Here's how the part is built. I have some questions about the finished solid (model axes, mm). A direction names the side the tool comes from. Give positions to 0.01 mm unless a question says otherwise; leave off trailing zeros. Loops run counter-clockwise (first coordinate to the right, second up) from the corner with the lowest first, then second, coordinate; pieces in that order, holes last.
Q1. Suppose I cut it at C-C (y = 219). List the corners of the cut face in (x, z) for me.
Q2. Suppose I cut it at D-D (z = 499). List the corners of the cut face in (x, y) for me.
Q3. Suppose I cut it at B-B (z = -166). List the corners of the cut face in (x, y) for me.
Q4. Thinking about a two-plate mould opening in X: for faces 6 (the face through (789.91, 959.68, -563.82)), 7 (the face through (-419.1, 161, -206)), 8 (the face through (201.28, 927.28, -543.77)), which applies, pulls with the +X half, pulls with the -X half, needs draft (parallel to the pull), parting line crosses it, or undercut?
Q5. I'm going to push flat-ended pins straight in: P1, Ø3, axis at x = -54, y = 900.5, coming from the +Z side; P2, Ø2, axis at x = 529.5, y = 641.5, coming from the +Z side; P3, Ø5, axis at x = 292, y = -83.5, coming from the -Z side. Where does each tip first touch, or does it pass through?
Q6. I need wall thicknesses on probe 1 along X at (y, z) = (108, -193.5); probe 2 along Y at (x, z) = (460.5, -430); probe 3 along X at (y, z) = (1042, -269.5). Which ranges of each line are inside material? Lowest first, please.
Q7. Suppose I cut it at A-A (x = 202.5). List the corners of the cut face in (y, z) for me, and give its area (3 significant figures).
Q8. For faces 1 (the face through (201.28, 456.34, -811.99)), 2 (the face through (790, 988.185, -258)), 3 (the face through (-266, 1123, -46.053)), 4 (the face through (201, 950.085, -263)), 5 (the face through (-372, 988.185, -258)), which set-ups out of +Z, -Z, +X, -X, +Y, -Y let a thin tool reach every point of the face, with its end or its side?
```python
from build123d import *

# Parameters (mm, degrees)
BOSS_EXTRUDE1_DEPTH = 419.1
SHELL1_START        = 12.7
SHELL1_DEPTH        = 393.7
BOSS_EXTRUDE3_START = -69.85
SKETCH3_R           = 12.7
BOSS_EXTRUDE3_DEPTH = 38.1
SCALE3_SCALE        = 3


# Read off the part's stored shape, not the designer's step: Shell1
with BuildPart() as part:
    # Sketch1 → Boss-Extrude1 (new body)
    with BuildSketch(Plane(origin=(0, 0, 0), x_dir=(0, 0, -1), z_dir=(1, 0, 0))):
        with BuildLine():
            Line((0, 0), (476.25, 0))
            ThreePointArc((476.25, 0), (564.93634732, 49.85994299), (568.425328349, 151.541352929))
            Line((568.425328349, 151.541352929), (428.331493685, 422.044080755))
            ThreePointArc((428.331493685, 422.044080755), (404.943942228, 447.093648811), (371.944875703, 456.341352929))
            Line((371.944875703, 456.341352929), (232.768876591, 456.341352929))
            Line((232.768876591, 456.341352929), (214.204669203, 445.076315348))
            Line((214.204669203, 445.076315348), (8.95741062, 50.8))
            Line((8.95741062, 50.8), (0, 0))
        make_face()
    extrude(amount=BOSS_EXTRUDE1_DEPTH)

    # Shell1 outline → Shell1 (cut)
    with BuildSketch(Plane.YZ.offset(SHELL1_START)):
        with BuildLine():
            Line((22.86, -4.030834779), (22.86, -434.440917972))
            ThreePointArc((22.86, -434.440917972), (39.418714995, -540.70503827), (145.700807364, -557.148004752))
            Line((145.700807364, -557.148004752), (416.20353519, -417.054170089))
            ThreePointArc((416.20353519, -417.054170089), (436.243189635, -398.344128923), (443.641352929, -371.944875703))
            Line((443.641352929, -371.944875703), (443.641352929, -236.320754436))
            Line((443.641352929, -236.320754436), (423.361553833, -202.900679848))
            Line((423.361553833, -202.900679848), (50.8, -8.95741062))
            Line((50.8, -8.95741062), (22.86, -4.030834779))
        make_face()
    extrude(amount=SHELL1_DEPTH, mode=Mode.SUBTRACT)

    # Sketch3 → Boss-Extrude3 (add)
    with BuildSketch(Plane(origin=(419.1, 0, 0), x_dir=(0, 0, -1), z_dir=(1, 0, 0)).offset(BOSS_EXTRUDE3_START)):
        with BuildLine():
            Line((232.768876591, 545.241352929), (232.768876591, 456.341352929))
            Line((232.768876591, 456.341352929), (371.944875703, 456.341352929))
            ThreePointArc((371.944875703, 456.341352929), (404.943942228, 447.093648811), (428.331493685, 422.044080755))
            Line((428.331493685, 422.044080755), (435.388694544, 408.417556164))
            Line((435.388694544, 408.417556164), (490.381307684, 440.167556164))
            ThreePointArc((490.381307684, 440.167556164), (496.298565678, 447.879076919), (495.029830312, 457.516078792))
            Line((495.029830312, 457.516078792), (482.329830312, 479.513124048))
            ThreePointArc((482.329830312, 479.513124048), (474.618309557, 485.430382042), (464.981307684, 484.161646676))
            Line((464.981307684, 484.161646676), (438.491684026, 468.867855326))
            Line((438.491684026, 468.867855326), (371.944875703, 500.791352929))
            Line((371.944875703, 500.791352929), (371.944875703, 545.241352929))
            ThreePointArc((371.944875703, 545.241352929), (368.225131824, 554.22160905), (359.244875703, 557.941352929))
            Line((359.244875703, 557.941352929), (245.468876591, 557.941352929))
            ThreePointArc((245.468876591, 557.941352929), (236.48862047, 554.22160905), (232.768876591, 545.241352929))
        make_face()
        with Locations((302.356876147, 532.541352929)):
            Circle(SKETCH3_R, mode=Mode.SUBTRACT)
        with Locations((466.682785056, 455.81460142)):
            Circle(SKETCH3_R, mode=Mode.SUBTRACT)
    boss_extrude3 = extrude(amount=BOSS_EXTRUDE3_DEPTH)

    # Mirror1: Boss-Extrude3 across plane
    add(boss_extrude3.mirror(Plane(origin=(209.55, 0, 0), x_dir=(0, 0, 1), z_dir=(1, 0, 0))))


with BuildPart() as part_1:
    # Scale3: scaled about (209.55, 190.419755822, -326.126976247)
    add(part.part.scale(SCALE3_SCALE).moved(Location((-419.1, -380.839511644, 652.253952494))))


solid = part_1.part
```
Solutions:
1. outline: (-419.1, -977.81) - (838.2, -977.81) - (838.2, 392.46) - (800.1, 392.46) - (800.1, -934.91) - (-381, -934.91) - (-381, 392.46) - (-419.1, 392.46) - close
2. outline: (-419.1, -380.84) - (838.2, -380.84) - (838.2, 14.34) - (800.1, 14.34) - (800.1, -312.26) - (-381, -312.26) - (-381, 14.34) - (-419.1, 14.34) - close
3. outline: (-419.1, -380.84) - (838.2, -380.84) - (838.2, 988.18) - (742.95, 988.18) - (742.95, 1292.98) - (628.65, 1292.98) - (628.65, 988.18) - (-209.55, 988.18) - (-209.55, 1292.98) - (-323.85, 1292.98) - (-323.85, 988.18) - (-419.1, 988.18) - close; hole (-381, -312.26) - (800.1, -312.26) - (800.1, 950.08) - (-381, 950.08) - close
4. face 6: needs draft
4. face 7: pulls with the -X half
4. face 8: undercut
5. P1: stops at z = 38.47
5. P2: stops at z = -715.58
5. P3: stops at z = -1087.69
6. probe 1: x = -419.1 to -381, 800.1 to 838.2
6. probe 2: y = -380.84 to -312.26, 950.08 to 988.18
6. probe 3: x = -323.85 to -209.55, 628.65 to 742.95
7. outline: (-380.84, -776.5) arc R311.41 ccw to (73.78, -1053.02) - (885.29, -632.74) arc R190.5 ccw to (988.18, -463.58) - (988.18, -46.05) - (954.39, 9.64) - (889.25, 43.55) - (950.08, -56.71) - (950.08, -463.58) arc R152.4 cw to (867.77, -598.91) - (56.26, -1019.19) arc R273.31 cw to (-312.26, -651.07) - (-312.26, 640.16) - (-380.84, 652.25) - close
7. area: 179,000 mm2
8. face 1: +Z
8. face 2: +Z, -Z, +X, +Y
8. face 3: +Z, +X, -X, +Y
8. face 4: none
8. face 5: +Z, -Z, -X, +Y
